from build123d import *

# Parameters (mm, degrees)
SKETCH1_W           = 100
SKETCH1_H           = 100
BOSS_EXTRUDE1_DEPTH = 80
SKETCH2_W           = 100
SKETCH2_H           = 100
BOSS_EXTRUDE2_DEPTH = 60
BOSS_EXTRUDE2_TAPER = 25
SKETCH3_W           = 100
SKETCH3_H           = 100
BOSS_EXTRUDE3_DEPTH = 60
BOSS_EXTRUDE3_TAPER = -35
SKETCH5_W           = 144.024904586
SKETCH5_H           = 144.024904586
CUT_EXTRUDE2_DEPTH  = 20
CUT_EXTRUDE2_TAPER  = -35
SKETCH6_W           = 30
SKETCH6_H           = 30
BOSS_EXTRUDE4_DEPTH = 20
DRAFT5_ANGLE        = 20


with BuildPart() as part:
    # Sketch1 → Boss-Extrude1 (new body)
    with BuildSketch(Plane(origin=(0, 0, 0), x_dir=(1, 0, 0), z_dir=(0, 1, 0))):
        Rectangle(SKETCH1_W, SKETCH1_H)
    extrude(amount=BOSS_EXTRUDE1_DEPTH)

    # Sketch2 → Boss-Extrude2 (add)
    with BuildSketch(Plane(origin=(0, 80, 0), x_dir=(1, 0, 0), z_dir=(0, 1, 0))):
        Rectangle(SKETCH2_W, SKETCH2_H)
    extrude(amount=BOSS_EXTRUDE2_DEPTH, taper=BOSS_EXTRUDE2_TAPER)

    # Sketch3 → Boss-Extrude3 (add)
    with BuildSketch(Plane.XZ):
        Rectangle(SKETCH3_W, SKETCH3_H)
    extrude(amount=BOSS_EXTRUDE3_DEPTH, taper=BOSS_EXTRUDE3_TAPER)

    # Sketch5 → Cut-Extrude2 (cut)
    with BuildSketch(Plane(origin=(0, -40, 0), x_dir=(-1, 0, 0), z_dir=(0, -1, 0))):
        Rectangle(SKETCH5_W, SKETCH5_H)
    extrude(amount=CUT_EXTRUDE2_DEPTH, taper=CUT_EXTRUDE2_TAPER, mode=Mode.SUBTRACT)

    # Sketch6 → Boss-Extrude4 (add)
    with BuildSketch(Plane(origin=(50, 0, 0), x_dir=(0, 0, -1), z_dir=(1, 0, 0))):
        with Locations((0, 40)):
            Rectangle(SKETCH6_W, SKETCH6_H)
    extrude(amount=BOSS_EXTRUDE4_DEPTH)

    # Draft5
    draft5_faces = [part.faces().sort_by_distance(p)[0] for p in [
        (60, 55, 0),
    ]]
    draft(draft5_faces, Plane(origin=(50, 80, 50), x_dir=(0, 0, 1), z_dir=(1, 0, 0)), DRAFT5_ANGLE)


solid = part.part
Here's how the part is built. I have some questions about the finished solid (model axes, mm). A direction names the side the tool comes from. Coordinates: 2 decimals unless noted, no trailing zeros. Order: outer loops, then holes, each group sorted by start corner. A loop starts at its lowest first (then second) coordinate and runs counter-clockwise, first axis right, second up. Notation, with made-up numbers: (25, 56) -> (83, 56) arc R17 ccw to (83, 78) -> close; hole circle Ø9 at (52.5, 65). An arc over 180 degrees is marked (long way). Answer in a Markdown table with one row per item.
(1) Thinking about a two-plate mould opening in Z: for faces 1 (the face through (2, -40, 0)), 2 (the face through (-89, -60, -7)), 3 (the face through (-1, 39, -50)), which applies, +Z half, -Z half, draft (parallel to the pull), parting line (faces both ways), or undercut?
Answer key:
| item | result |
|---|---|
| face 1 | undercut |
| face 2 | draft |
| face 3 | -Z half |
(2) Please list where these lines run through material, in increasing order: probe 1 along Y at (x, z) = (1.5, -14.5); probe 2 along X at (y, z) = (58, 24.5); probe 3 along Z at (x, y) = (-66, -42).
Answer key:
| item | result |
|---|---|
| probe 1 | -40 to 140 |
| probe 2 | -50 to 50 |
| probe 3 | -79.41 to -73.41, 73.41 to 79.41 |
(3) On a 3-axis mill with a long thin cutter (end or side, diameter ignored), from which of +Z, -Z, +X, -X, +Y, -Y can I reach the whole of each face in a straight line? I mean faces 4 (the face through (70, 37, 0)), 5 (the face through (60, 40, -15)), 6 (the face through (-50, 39, 1)), 7 (the face through (60, 25, 0)). Say none if no direction works.
Answer key:
| item | result |
|---|---|
| face 4 | +Z, -Z, +X, +Y |
| face 5 | -Z, +X, +Y |
| face 6 | +Z, -Z, -X, +Y |
| face 7 | +Z, -Z, +X |
(4) I want a section at A-A on y = 9. List the corners of the cut face in (x, z) for me, then the cut area to 3 significant figures.
Answer key:
| item | result |
|---|---|
| outline | (-50, -50) -> (50, -50) -> (50, 50) -> (-50, 50) -> close |
| area | 10,000 mm^2 |
(5) Will these pins go through, and if not, where does the flat tip stop? pin 1 Ø24 at (x, y) = (-18.5, 32) entering from +Z; pin 2 Ø22 at (x, y) = (63, 44.5) entering from -Z; pin 3 Ø1 at (y, z) = (-27, 53.5) entering from -X.
Answer key:
| item | result |
|---|---|
| pin 1 | z = 50 |
| pin 2 | z = -15 |
| pin 3 | x = -69.26 |
